from build123d import *

# Parameters (mm, degrees)
CYLINDER969_R     = 74
CYLINDER969_DEPTH = 40
BOX480_W          = 50
BOX480_H          = 6
BOX480_DEPTH      = 26
CHAMFER011_SIZE   = 20


with BuildPart() as obj1:
    # Cylinder969 → Cylinder969 (new body)
    with BuildSketch(Plane.XY.offset(42)):
        Circle(CYLINDER969_R)
    extrude(amount=CYLINDER969_DEPTH)


with BuildPart() as chamfer011:
    # Box480 → Box480 (new body)
    with BuildSketch(Plane(origin=(3, -112, 56), x_dir=(0, 1, 0), z_dir=(0, 0, 1))):
        with Locations((25, 3)):
            Rectangle(BOX480_W, BOX480_H)
    extrude(amount=BOX480_DEPTH)

    # Cut449: cut obj1
    add(obj1.part, mode=Mode.SUBTRACT)

    # Chamfer011
    chamfer011_edges = [chamfer011.edges().sort_by_distance(p)[0] for p in [
        (0, -112, 56),
    ]]
    chamfer(chamfer011_edges, length=CHAMFER011_SIZE)


solid = chamfer011.part
The listing builds one solid part. Answer for the finished solid, in the listing's coordinates (mm). Round coordinates to 2 decimals unless told otherwise and drop trailing zeros. Write each loop counter-clockwise with the first axis right and the second up, starting at its lowest first coordinate (ties: lowest second). Pieces come first, ordered by that corner, then holes. Notation, with made-up numbers: M -36,80 L -19,80 A36 ccw -19,118 Z; hole C 12,34.25 d10. An arc over 180 degrees is marked long. Write each question's results on one line, items separated by ' | '. Start each with the question number.
Item 1: Given pin 1 Ø1 at (x, y) = (2.5, -101.5) entering from -Z; pin 2 Ø6 at (y, z) = (-107, 63) entering from -X, each flat-ended and moving along its own axis, determine where each tip first touches the part or whether it passes through.
Item 2: The mould has two halves that part along X. Classify faces 1 (the flat face through (-3, -89, 72)), 2 (the flat face through (0, -112, 79)), 3 (the cylindrical face through (0, -74, 69)): +X half, -X half, draft (parallel to the pull), parting line (faces both ways), or undercut.
Item 3: Find section B-B on y = -107.5. Write down the section's boundary in (x, z), and give its area (3 significant figures).
Item 4: Find section D-D on x = -0.5. Write down the section's boundary in (y, z).
Item 5: Find section C-C on x = 1.75. Write down the section's boundary in (y, z), and give its area (3 significant figures).
Item 6: Straight lines are drawn through the part: probe 1 along Y at (x, z) = (0.5, 79); probe 2 along Z at (x, y) = (1, -108); probe 3 along Y at (x, z) = (0.5, 66.25). For each, find the intervals that lie inside material, in ascending order.
Item 7: Find section A-A on z = 66.5. Write down the section's boundary in (x, y).
Answer block:
1) pin 1: stops at z = 65 | pin 2: passes through
2) face 1: -X half | face 2: draft | face 3: undercut
3) outline: M -3,71.5 L 3,71.5 L 3,82 L -3,82 Z | area: 63.0 mm²
4) outline: M -112,76 L -92,56 L -74,56 L -74,82 L -112,82 Z
5) outline: M -112,76 L -92,56 L -73.98,56 L -73.98,82 L -112,82 Z | area: 789 mm²
6) probe 1: y = -112 to -74 | probe 2: z = 72 to 82 | probe 3: y = -102.25 to -74
7) outline: M -3,-102.5 L 3,-102.5 L 3,-73.94 A74 cw -3,-73.94 Z
